The listing builds one solid part. Answer for the finished solid, in the listing's coordinates (mm). Face numbers are marked on the shaded views. A direction names the side the tool comes from. Give positions to 0.01 mm unless a question says otherwise; leave off trailing zeros. Write each loop counter-clockwise with the first axis right and the second up, starting at its lowest first coordinate (ties: lowest second). Pieces come first, ordered by that corner, then holes. Notation, with made-up numbers: (60, 52) -> (111, 52) arc R21 cw to (111, 71) -> close; hole circle Ø1 at (79.5, -31.5). An arc over 180 degrees is marked (long way). Put each result on its own line as item: value. Start each with the question number.
1) Find the intervals of material crossed by line 1 along Y through (x, z) = (-8.5, 11.75); line 2 along Z through (x, y) = (-14.5, 10); line 3 along X through (y, z) = (19.5, 14.75), in increasing order. Write a range as from..to.
2) A cutting plane is placed at D-D (z = 15). Write down the section's boundary in (x, y), then the cut area to 3 significant figures.
3) For the marked faces 4, 5, 6 and 7, determine the directions among +Z, -Z, +X, -X, +Y, -Y from which every point of the face is accessible in a straight line to the end or side of a thin tool.
4) For a pull along X with two mould halves and no side action, classify the marked faces 1, 2 and 3 as released by +X, released by -X, zero draft, split by the parting line, or undercut.
5) A cutting plane is placed at B-B (z = 9). Write down the section's boundary in (x, y), then the cut area to 3 significant figures.
6) Flat-ended cylindrical pins translate along their axes: pin 1 Ø6 at (x, y) = (-12.5, 3) entering from -Z; pin 2 Ø3 at (y, z) = (44.5, 14) entering from +X; pin 3 Ø1.8 at (x, z) = (3, 12.5) entering from -Y; pin 4 Ø4 at (x, z) = (-3.5, 12) entering from +Y. Find the tip coordinate at first contact, or state that the pin passes through.
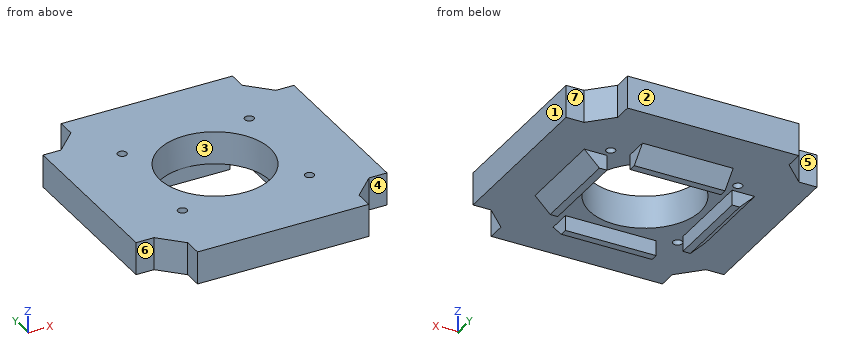
Autodesk Inventor part; units mm, degrees
ref_plane "Work Plane1" through (0, 0, 10) normal (0, 0, 1) x (1, 0, 0)
ref_plane "Work Plane2" through (-40.9959, 0.8639, 22.2359) normal (0, 0, 1) x (1, 0, 0)
ref_plane "YZ Plane" through (0, 0, 0) normal (1, 0, 0) x (0, 1, 0)
ref_plane "Work Plane1" through (0, 0, 10) normal (0, 0, 1) x (1, 0, 0)
sketch "Sketch1" plane through (0, 0, 10) normal (0, 0, 1) x (1, 0, 0)
  line L0 (-4.0299, -0.3538) -> (-2.2322, 1.4439) construction
  arc A0 (-1.4439, 2.2322) -> (-2.2322, 1.4439) centre (-0.9299, 0.9299) ccw construction
  line L1 (-1.4439, 2.2322) -> (0.3538, 4.0299) construction
  line L2 (-37.8299, 42.2137) -> (-37.8299, 45.8299) construction
  line L3 (-37.8299, 45.8299) -> (-4.0299, 45.8299) construction
  line L4 (-4.0299, 45.8299) -> (-4.0299, 42.2137) construction
  line L5 (-4.0299, 4.0299) -> (0.3538, 4.0299)
  line L6 (-20.9299, 58.9723) -> (17.1124, 20.9299) construction
  line L7 (17.1124, 20.9299) -> (-20.9299, -17.1124) construction
  line L8 (-20.9299, -17.1124) -> (-58.9723, 20.9299) construction
  line L9 (-58.9723, 20.9299) -> (-20.9299, 58.9723) construction
  line L10 (-20.9299, 58.9723) -> (-20.9299, -17.1124) construction
  line L11 (17.1124, 20.9299) -> (-58.9723, 20.9299) construction
  line L12 (-20.9299, 58.9723) -> (32.8701, 58.9723) construction
  line L13 (-43.4299, 43.4299) -> (1.5701, 43.4299) construction
  line L14 (1.5701, 43.4299) -> (1.5701, -1.5701) construction
  line L15 (1.5701, -1.5701) -> (-43.4299, -1.5701) construction
  line L16 (-43.4299, -1.5701) -> (-43.4299, 43.4299) construction
  line L17 (-43.4299, 43.4299) -> (1.5701, -1.5701) construction
  line L18 (1.5701, 43.4299) -> (-43.4299, -1.5701) construction
  line L19 (-43.4299, 5.3876) -> (-43.4299, 36.4723)
  line L20 (-43.4299, 36.4723) -> (-36.4723, 43.4299)
  line L21 (-36.4723, 43.4299) -> (-5.3876, 43.4299)
  line L22 (-5.3876, 43.4299) -> (1.5701, 36.4723)
  line L23 (1.5701, 36.4723) -> (1.5701, 5.3876)
  line L24 (1.5701, 5.3876) -> (-5.3876, -1.5701)
  line L25 (-5.3876, -1.5701) -> (-36.4723, -1.5701)
  line L26 (-36.4723, -1.5701) -> (-43.4299, 5.3876)
  line L27 (-4.0299, 42.2137) -> (-37.8299, 42.2137)
  line L28 (-4.0299, -0.3538) -> (-4.0299, 4.0299)
  circle A1 centre (-20.9299, 20.9299) radius 13.3985
  circle A2 centre (-20.9299, 20.9299) radius 15.4895
  point P0 (-37.8299, 4.0299)
  dimension "d18" = 53.8
  dimension "d19" = 45
  dimension "d20" = 53.8
  dimension "d21" = 45
  dimension "d22" = 45
  dimension "d30" = 26.797
  dimension "d36" = 30.979
extrude "Extrusion1" add sketch "Sketch1" along normal blind 6.5 contours L28 L24 L25 L26 L19 L20 L27 L22 L23 L5 | L5 L24 L28 | L27 L20 L21 L22 | A1 | A2
ref_plane "Work Plane2" through (-40.9959, 0.8639, 22.2359) normal (0, 0, 1) x (1, 0, 0)
sketch "Sketch3" plane through (0, 0, 10) normal (0, 0, -1) x (-1, 0, 0)
  line L0 (37.8299, -0.4701) -> (37.8299, 4.0299) construction
  line L1 (4.0299, 4.0299) -> (4.0299, -0.4701) construction
  line L2 (37.8299, -0.4701) -> (37.8299, 1.1886) construction
  line L3 (4.0299, -3.9701) -> (4.0299, -0.3538) construction
  line L4 (45.8299, 4.0299) -> (42.2137, 4.0299) construction
  line L5 (-0.3538, 4.0299) -> (-3.9701, 4.0299) construction
  line L6 (-3.9701, 37.8299) -> (-0.3538, 37.8299) construction
  line L7 (4.0299, 42.2137) -> (4.0299, 45.8299) construction
  line L8 (37.8299, 45.8299) -> (37.8299, 42.2137) construction
  line L9 (42.2137, 37.8299) -> (45.8299, 37.8299) construction
  line L10 (37.8299, 37.7299) -> (45.8299, 37.7299)
  line L11 (45.8299, 37.7299) -> (45.8299, 4.1299)
  line L12 (45.8299, 4.1299) -> (37.8299, 4.1299)
  line L13 (37.8299, 4.1299) -> (37.8299, 37.7299)
  line L14 (37.7299, 4.0299) -> (4.1299, 4.0299)
  line L15 (4.1299, 4.0299) -> (4.1299, -3.9701)
  line L16 (4.1299, -3.9701) -> (37.7299, -3.9701)
  line L17 (37.7299, -3.9701) -> (37.7299, 4.0299)
  line L18 (4.0299, 4.1299) -> (-3.9701, 4.1299)
  line L19 (-3.9701, 4.1299) -> (-3.9701, 37.7299)
  line L20 (-3.9701, 37.7299) -> (4.0299, 37.7299)
  line L21 (4.0299, 37.7299) -> (4.0299, 4.1299)
  line L22 (4.1299, 37.8299) -> (37.7299, 37.8299)
  line L23 (37.7299, 37.8299) -> (37.7299, 45.8299)
  line L24 (37.7299, 45.8299) -> (4.1299, 45.8299)
  line L25 (4.1299, 45.8299) -> (4.1299, 37.8299)
  point P0 (0, 0)
  dimension "d23" = 0.1
  dimension "d24" = 0.1
  dimension "d25" = 0.1
  dimension "d26" = 0.1
  dimension "d27" = 0.1
extrude "Extrusion3" add sketch "Sketch3" against normal up to surface (6.5 mm away)
sketch "Sketch6" plane through (0, 0, 16.5) normal (0, 0, 1) x (1, 0, 0)
  circle A0 centre (-20.9299, 20.9299) radius 15.4895
  circle A1 centre (-20.9299, 20.9299) radius 11
  line L0 (-45.8299, 4.1299) -> (-45.8299, 37.7299)
  line L1 (-4.1299, -3.9701) -> (-37.7299, -3.9701)
  line L2 (-37.7299, 45.8299) -> (-4.1299, 45.8299)
  point P0 (0, 0)
  point P1 (-45.8299, 20.9299)
  point P2 (-20.9299, -3.9701)
  point P3 (-20.9299, 45.8299)
  dimension "d37" = 22
  dimension "d38" = 30.979
extrude "Extrusion5" cut sketch "Sketch6" against normal blind 12 contours A1
sketch "Skizze12" plane through (0, 0, 16.5) normal (0, 0, 1) x (1, 0, 0)
  circle A0 centre (-20.9299, 20.9299) radius 11 construction
  line L0 (3.9701, 4.1299) -> (0.3124, 4.1299)
  line L1 (3.9701, 37.7299) -> (3.9701, 4.1299) construction
  line L2 (0.3124, 37.7299) -> (3.9701, 37.7299)
  line L3 (0.3124, 37.7299) -> (-4.1299, 42.1723)
  line L4 (-4.1299, 45.8299) -> (-4.1299, 42.1723)
  line L5 (-37.7299, 45.8299) -> (-4.1299, 45.8299) construction
  line L6 (-37.7299, 42.1723) -> (-37.7299, 45.8299)
  line L7 (-37.7299, 42.1723) -> (-42.1723, 37.7299)
  line L8 (-45.8299, 37.7299) -> (-42.1723, 37.7299)
  line L9 (-45.8299, 4.1299) -> (-45.8299, 37.7299) construction
  line L10 (-42.1723, 4.1299) -> (-45.8299, 4.1299)
  line L11 (-42.1723, 4.1299) -> (-37.7299, -0.3124)
  line L12 (-37.7299, -3.9701) -> (-37.7299, -0.3124)
  line L13 (-4.1299, -3.9701) -> (-37.7299, -3.9701) construction
  line L14 (-4.1299, -0.3124) -> (-4.1299, -3.9701)
  line L15 (-4.1299, -0.3124) -> (0.3124, 4.1299)
  line L16 (-3.9299, 46.0299) -> (-3.9299, 42.2551)
  line L17 (-3.9299, 42.2551) -> (0.3953, 37.9299)
  line L18 (0.3953, 37.9299) -> (4.1701, 37.9299)
  line L19 (4.1701, 37.9299) -> (4.1701, 3.9299) construction
  line L20 (4.1701, 3.9299) -> (0.3953, 3.9299)
  line L21 (0.3953, 3.9299) -> (-3.9299, -0.3953)
  line L22 (-3.9299, -0.3953) -> (-3.9299, -4.1701)
  line L23 (-3.9299, -4.1701) -> (-37.9299, -4.1701) construction
  line L24 (-37.9299, -4.1701) -> (-37.9299, -0.3953)
  line L25 (-37.9299, -0.3953) -> (-42.2551, 3.9299)
  line L26 (-42.2551, 3.9299) -> (-46.0299, 3.9299)
  line L27 (-46.0299, 3.9299) -> (-46.0299, 37.9299) construction
  line L28 (-46.0299, 37.9299) -> (-42.2551, 37.9299)
  line L29 (-42.2551, 37.9299) -> (-37.9299, 42.2551)
  line L30 (-37.9299, 42.2551) -> (-37.9299, 46.0299)
  line L31 (-37.9299, 46.0299) -> (-3.9299, 46.0299) construction
  line L32 (-45.8299, 37.7299) -> (-45.8299, 37.9299)
  line L33 (-37.7299, 45.8299) -> (-37.9299, 45.8299)
  line L34 (-4.1299, 45.8299) -> (-3.9299, 45.8299)
  line L35 (3.9701, 37.7299) -> (3.9701, 37.9299)
  line L36 (3.9701, 4.1299) -> (0.3124, 4.1299)
  line L37 (3.9701, 4.1299) -> (3.9701, 3.9299)
  line L38 (-4.1299, -3.9701) -> (-3.9299, -3.9701)
  line L39 (-37.7299, -3.9701) -> (-37.9299, -3.9701)
  line L40 (-45.8299, 4.1299) -> (-45.8299, 3.9299)
  point P0 (0, 0)
  dimension "d93" = 0.2
extrude "IM_offset" add sketch "Skizze12" against normal up to surface (6.5 mm away)
sketch "Sketch13" plane through (0, 0, 10) normal (0, 0, -1) x (-1, 0, 0)
  arc A0 (8.6799, 30.7299) -> (8.6799, 32.7299) centre (8.6799, 31.7299) ccw
  arc A1 (33.1799, 32.7299) -> (33.1799, 30.7299) centre (33.1799, 31.7299) ccw
  arc A2 (33.1799, 10.7299) -> (33.1799, 8.7299) centre (33.1799, 9.7299) ccw
  arc A3 (8.6799, 8.7299) -> (8.6799, 10.7299) centre (8.6799, 9.7299) ccw
  circle A4 centre (8.258, 9.7299) radius 0.9
  circle A5 centre (8.258, 31.7299) radius 0.9
  circle A6 centre (33.4928, 31.7299) radius 0.9
  circle A7 centre (33.4928, 9.7299) radius 0.9
  point P0 (0, 0)
  dimension "d96" = 1.8
  dimension "d97" = 1.8
  dimension "d98" = 1.8
  dimension "d99" = 1.8
extrude "Extrusion9" cut sketch "Sketch13" against normal blind 10
sketch "Sketch14" plane through (0, 0, 10) normal (0, 0, -1) x (-1, 0, 0)
  circle A0 centre (20.9299, 20.9299) radius 11
  line L0 (29.9299, 32.0648) -> (11.9299, 32.0648)
  line L1 (11.9299, 32.0648) -> (11.9299, 33.5648)
  line L2 (11.9299, 33.5648) -> (29.9299, 33.5648)
  line L3 (29.9299, 33.5648) -> (29.9299, 32.0648)
  line L4 (29.9299, 32.0648) -> (11.9299, 33.5648) construction
  line L5 (11.9299, 32.0648) -> (29.9299, 33.5648) construction
  line L6 (29.9299, 6.9335) -> (11.9299, 6.9335)
  line L7 (11.9299, 6.9335) -> (11.9299, 8.4335)
  line L8 (11.9299, 8.4335) -> (29.9299, 8.4335)
  line L9 (29.9299, 8.4335) -> (29.9299, 6.9335)
  line L10 (29.9299, 6.9335) -> (11.9299, 8.4335) construction
  line L11 (11.9299, 6.9335) -> (29.9299, 8.4335) construction
  line L12 (6.9935, 29.9299) -> (8.4935, 29.9299)
  line L13 (8.4935, 29.9299) -> (8.4935, 11.9299)
  line L14 (8.4935, 11.9299) -> (6.9935, 11.9299)
  line L15 (6.9935, 11.9299) -> (6.9935, 29.9299)
  line L16 (6.9935, 29.9299) -> (8.4935, 11.9299) construction
  line L17 (8.4935, 29.9299) -> (6.9935, 11.9299) construction
  line L18 (33.3254, 29.9299) -> (34.8254, 29.9299)
  line L19 (34.8254, 29.9299) -> (34.8254, 11.9299)
  line L20 (34.8254, 11.9299) -> (33.3254, 11.9299)
  line L21 (33.3254, 11.9299) -> (33.3254, 29.9299)
  line L22 (33.3254, 29.9299) -> (34.8254, 11.9299) construction
  line L23 (34.8254, 29.9299) -> (33.3254, 11.9299) construction
  point P0 (0, 0)
  point P1 (20.9299, 32.8148)
  point P2 (20.9299, 7.6835)
  point P3 (7.7435, 20.9299)
  point P4 (34.0754, 20.9299)
  dimension "d102" = 18
  dimension "d103" = 1.5
  dimension "d104" = 1.5
  dimension "d105" = 1.5
  dimension "d106" = 18
  dimension "d107" = 1.5
  dimension "d108" = 18
extrude "Extrusion10" add sketch "Sketch14" along normal blind 3 contours L0 L1 L2 L3 | L6 L7 L8 L9 | L12 L13 L14 L15 | L18 L19 L20 L21
chamfer "Chamfer1" distance 3 angle 45 4 edges at (-20.9299, 6.9335, 10) (-6.9935, 20.9299, 10) (-20.9299, 33.5648, 10) (-34.8254, 20.9299, 10)
properties part number "20_Cube_Insert_Laser_Holder_fixed_v3"
Reply:
1. line 1: y = -3.97..8.86, 10.6..30.86, 32.6..45.83
1. line 2: z = 10..16.5
1. line 3: x = -45.83..-31.84, -10.02..3.97
2. outline: (-45.83, 3.93) -> (-42.26, 3.93) -> (-37.93, -0.4) -> (-37.93, -3.97) -> (-3.93, -3.97) -> (-3.93, -0.4) -> (0.4, 3.93) -> (3.97, 3.93) -> (3.97, 37.93) -> (0.4, 37.93) -> (-3.93, 42.26) -> (-3.93, 45.83) -> (-37.93, 45.83) -> (-37.93, 42.26) -> (-42.26, 37.93) -> (-45.83, 37.93) -> close; hole circle Ø1.8 at (-33.49, 9.73); hole circle Ø1.8 at (-33.49, 31.73); hole circle Ø22 at (-20.93, 20.93); hole circle Ø1.8 at (-8.26, 9.73); hole circle Ø1.8 at (-8.26, 31.73)
2. area: 1,880 mm2
3. face 4: +Z, -Z, +X, -Y
3. face 5: +Z, -Z, -X, +Y
3. face 6: +Z, -Z, -X, -Y
3. face 7: +Z, -Z, +X, +Y
4. face 1: released by +X
4. face 2: zero draft
4. face 3: undercut
5. outline: (-36.83, 11.93) -> (-33.33, 11.93) -> (-33.33, 29.93) -> (-36.83, 29.93) -> close; (-29.93, 4.93) -> (-11.93, 4.93) -> (-11.93, 8.43) -> (-29.93, 8.43) -> close; (-29.93, 32.06) -> (-11.93, 32.06) -> (-11.93, 35.56) -> (-29.93, 35.56) -> close; (-8.49, 11.93) -> (-4.99, 11.93) -> (-4.99, 29.93) -> (-8.49, 29.93) -> close
5. area: 252 mm2
6. pin 1: stops at z = 7.93
6. pin 2: stops at x = -3.93
6. pin 3: stops at y = 3.93
6. pin 4: stops at y = 45.83
